```python
from build123d import *

# Parameters (mm, degrees)
F0_R     = 17.5
F1_DEPTH = 25


with BuildPart() as f1:
    # F0 (on Front) → F1 (new body)
    with BuildSketch(Plane.XZ):
        with BuildLine():
            Line((47.495888, 15.625), (35.621916, 51.71875))
            ThreePointArc((35.621916, 51.71875), (0, 77.5), (-35.621916, 51.71875))
            Line((-35.621916, 51.71875), (-47.495888, 15.625))
            ThreePointArc((-47.495888, 15.625), (0, -50), (47.495888, 15.625))
        make_face()
        Circle(F0_R, mode=Mode.SUBTRACT)
    extrude(amount=F1_DEPTH)


solid = f1.part
```
Geometry check sheet. Reference: the model listing, model coordinates, mm. Round coordinates to 2 decimals unless told otherwise and drop trailing zeros. Order: outer loops, then holes, each group sorted by start corner. A loop starts at its lowest first (then second) coordinate and runs counter-clockwise, first axis right, second up. Notation, with made-up numbers: M 68,34 L 99,34 A24 cw 99,57 Z; hole C 12,-22 d8. An arc over 180 degrees is marked long. Answer as CSV lines item,"result".
1) Sectioned sample at B-B on x = 0. Record the cut outline in (y, z).
Entries:
outline,"M -25,-50 L 0,-50 L 0,-17.5 L -25,-17.5 Z; M -25,17.5 L 0,17.5 L 0,77.5 L -25,77.5 Z"
2) Mould release check, pull along X, two halves, no side actions. Record for faces 1 (the face through (10, -25, 15)), 2 (the face through (-13.887, -12.325, -10.648)), 3 (the face through (0.658, -12.325, 77.494)): +X half, -X half, draft (parallel to the pull), parting line (faces both ways), or undercut.
Entries:
face 1,"draft"
face 2,"undercut"
face 3,"parting line"
3) Sectioned sample at C-C on y = -15. Record the cut outline in (x, z) (3 decimals).
Entries:
outline,"M -47.496,15.625 A50 ccw long 47.496,15.625 L 35.622,51.719 A37.5 ccw -35.622,51.719 Z; hole C 0,0 d35"
4) Gauge pin test, flat ends, axial feed: pin 1 Ø10 at (y, z) = (-22, -7) entering from -X; pin 2 Ø10 at (x, y) = (34.5, -22.5) entering from +Z; pin 3 Ø2 at (x, y) = (-14, -20) entering from -Z. Record the tip position at first contact, or that the pin passes through.
Entries:
pin 1,"x = -49.96"
pin 2,"z = 63.15"
pin 3,"z = -48.28"
5) Thickness scan on probe 1 along Z at (x, y) = (0, -20); probe 2 along Z at (x, y) = (14.5, -12); probe 3 along X at (y, z) = (-17, 64.5). Record the ranges inside material, lowest first. Write a range as [from, to].
Entries:
probe 1,"[-50, -17.5], [17.5, 77.5]"
probe 2,"[-47.85, -9.8], [9.8, 74.58]"
probe 3,"[-28.39, 28.39]"
6) Sectioned sample at D-D on z = 34.5. Record the cut outline in (x, y).
Entries:
outline,"M -41.29,-25 L 41.29,-25 L 41.29,0 L -41.29,0 Z"
7) Sectioned sample at A-A on z = 0. Record the cut outline in (x, y), and give its area (4 significant figures).
Entries:
outline,"M -50,-25 L -17.5,-25 L -17.5,0 L -50,0 Z; M 17.5,-25 L 50,-25 L 50,0 L 17.5,0 Z"
area,"1,625 mm2"
